Geometry: final body of the model. Coordinates: model frame, mm. Round coordinates to 2 decimals unless told otherwise and drop trailing zeros. Loops run counter-clockwise (first coordinate to the right, second up) from the corner with the lowest first, then second, coordinate; pieces in that order, holes last. Notation, with made-up numbers: M 12,2.5 L 58,2.5 A16 cw 58,23.5 Z; hole C 66,-16 d11. An arc over 180 degrees is marked long. Answer as a JSON object with one key per item and string values.
Autodesk Inventor part; units mm, degrees
ref_plane "Work Plane1" through (0, 2, 0) normal (0, 1, 0) x (1, 0, 0)
ref_plane "YZ Plane" through (0, 0, 0) normal (1, 0, 0) x (0, 1, 0)
ref_plane "XZ Plane" through (0, 0, 0) normal (0, 1, 0) x (-1, 0, 0)
sketch "Sketch1" plane through (0, 0, 0) normal (0, 1, 0) x (-1, 0, 0)
  circle A0 centre (0, 0) radius 3.5005
  circle A1 centre (0, 0) radius 2.5
  dimension "d0" = 7.001
  dimension "d1" = 5.0001
extrude "Extrusion1" add sketch "Sketch1" along normal blind 2
ref_plane "Work Plane1" through (0, 2, 0) normal (0, 1, 0) x (1, 0, 0)
sketch "Sketch2" plane through (0, 2, 0) normal (0, 1, 0) x (1, 0, 0)
  arc A0 (0.2288, 3.4855) -> (0.2265, -3.4856) centre (0, 0) ccw
  arc A1 (16.1589, -2.4501) -> (16.1605, 2.4395) centre (16, -0.0053) ccw
  circle A2 centre (0, 0) radius 3.5005
  line L0 (0, 3.5005) -> (16.1605, 2.4395)
  line L1 (16.1589, -2.4501) -> (0.2265, -3.4856)
  circle A3 centre (0, 0) radius 2.5
  circle A4 centre (0, 0) radius 2.5
  dimension "d5" = 4.9
  dimension "d6" = 16
extrude "Extrusion2" add sketch "Sketch2" along normal blind 2.5 contours L0 A2 L1 A0 | A0 L1 A2 L0 | L0 A1 L1 A2
properties part number "eje de motor"
1) Line query: probe 1 along X at (y, z) = (3.2, 0); probe 2 along Z at (x, y) = (0, 2.55); probe 3 along Y at (x, z) = (7, -0.25). Output: solid intervals per line, ascending.
Geometry results:
{"probe 1": "-3.5 to -2.5, 2.5 to 18.45", "probe 2": "-3.5 to -2.5, 2.5 to 3.5", "probe 3": "2 to 4.5"}
2) Pull-direction query (X, two-part tool) for faces 1 (the face through (0.165, 2.218, 2.495)), 2 (the face through (-3.07, 2.22, 1.68)), 3 (the face through (18.45, 3.23, -0.05)); classes: +X half, -X half, draft (parallel to the pull), parting line (faces both ways), or undercut.
Geometry results:
{"face 1": "undercut", "face 2": "parting line", "face 3": "+X half"}
3) First-contact query: pin 1 (2 mm diameter, centred on y = 3.5, z = -2, fed in from +X); pin 2 (1.5 mm diameter, centred on x = 5.5, z = -1.5, fed in from -Y). Flat tips, straight axial feed; report the tip coordinate or a pass-through.
Geometry results:
{"pin 1": "x = 18.23", "pin 2": "y = 2"}
4) Cut plane A-A on y = 0.75. Return the cut outline in (x, z), and give its area (3 significant figures).
Geometry results:
{"outline": "C 0,0 d7; hole C 0,0 d5", "area": "18.9 mm2"}
5) Cut plane C-C on z = -3. Return the cut outline in (x, y), and give its area (3 significant figures).
Geometry results:
{"outline": "M -1.8,0 L 1.8,0 L 1.8,2 L 7.62,2 L 7.62,4.5 L -1.8,4.5 Z", "area": "30.8 mm2"}
6) Cut plane D-D on x = 15. Return the cut outline in (y, z).
Geometry results:
{"outline": "M 2,-2.52 L 4.5,-2.52 L 4.5,2.53 L 2,2.53 Z"}
